Source: CAD feature listing. Evaluate the final solid. Frame: model axes, mm. Face numbers are marked on the shaded views. Give positions to 0.01 mm unless a question says otherwise; leave off trailing zeros. Order: outer loops, then holes, each group sorted by start corner. A loop starts at its lowest first (then second) coordinate and runs counter-clockwise, first axis right, second up. Notation, with made-up numbers: (10, -4.75) -> (20, -4.75) arc R21 cw to (20, 4.25) -> close; hole circle Ø4 at (-36, 58.5). An arc over 180 degrees is marked (long way). Answer in a Markdown table with one row per item.
```python
from build123d import *

# Parameters (mm, degrees)
BOSS_EXTRUDE1_DEPTH = 20
SKETCH2_R           = 10
CUT_EXTRUDE1_DEPTH  = 20


with BuildPart() as part:
    # Sketch1 → Boss-Extrude1 (new body)
    with BuildSketch(Plane.XY):
        Polygon((-19.976319314, 0), (-9.988159657, -17.3), (9.988159657, -17.3), (19.976319314, 0), (9.988159657, 17.3), (-9.988159657, 17.3), align=None)
    extrude(amount=BOSS_EXTRUDE1_DEPTH)

    # Sketch2 → Cut-Extrude1 (cut)
    with BuildSketch(Plane.XY.offset(20)):
        Circle(SKETCH2_R)
    extrude(amount=-CUT_EXTRUDE1_DEPTH, mode=Mode.SUBTRACT)

    # Sketch3 → Cut-Revolve1 (revolve, cut)
    with BuildSketch(Plane(origin=(0, 0, 0), x_dir=(1, 0, 0), z_dir=(0, 1, 0))):
        with BuildLine():
            Line((19.976319314, -2), (19.976319314, 0))
            Line((19.976319314, 0), (17.976319314, 0))
            ThreePointArc((17.976319314, 0), (19.390532876, -0.585786438), (19.976319314, -2))
        make_face()
    cut_revolve1 = revolve(axis=Axis((0, 0, 0), (0, 0, 1)), mode=Mode.SUBTRACT)

    # Mirror1: Cut-Revolve1 across plane
    add(cut_revolve1.mirror(Plane(origin=(0, 0, 10), x_dir=(1, 0, 0), z_dir=(0, 0, -1))), mode=Mode.SUBTRACT)


solid = part.part
```
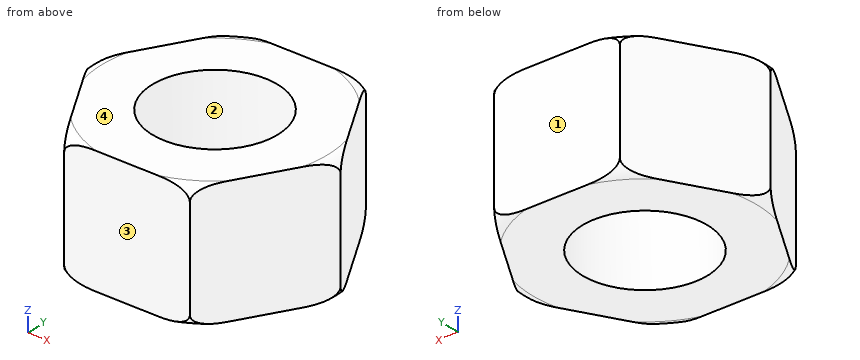
(1) Ray query, probe 1 along Y at (x, z) = (0, 14); probe 2 along Y at (x, z) = (-8.5, 6); probe 3 along X at (y, z) = (-4.5, 9.25). Return the intervals inside material, ascending.
A:
| item | result |
|---|---|
| probe 1 | y = -17.3 to -10, 10 to 17.3 |
| probe 2 | y = -17.3 to -5.27, 5.27 to 17.3 |
| probe 3 | x = -17.38 to -8.93, 8.93 to 17.38 |
(2) Section query D-D (z = 18.5). Return the cut outline in (x, y), plus the area to 3 significant figures.
A:
| item | result |
|---|---|
| outline | (-19.91, -0.11) -> (-10.05, -17.19) arc R19.91 ccw to (-9.86, -17.3) -> (9.86, -17.3) arc R19.91 ccw to (10.05, -17.19) -> (19.91, -0.11) arc R19.91 ccw to (19.91, 0.11) -> (10.05, 17.19) arc R19.91 ccw to (9.86, 17.3) -> (-9.86, 17.3) arc R19.91 ccw to (-10.05, 17.19) -> (-19.91, 0.11) arc R19.91 ccw to start; hole circle Ø20 at (0, 0) |
| area | 723 mm^2 |
(3) Pull-direction query (Y, two-part tool) for the marked faces 1, 2, 3 and 4; classes: +Y half, -Y half, draft (parallel to the pull), parting line (faces both ways), or undercut.
A:
| item | result |
|---|---|
| face 1 | +Y half |
| face 2 | undercut |
| face 3 | -Y half |
| face 4 | draft |
(4) Section query A-A (x = 0). Return the cut outline in (y, z).
A:
| item | result |
|---|---|
| outline | (-17.3, 0) -> (-10, 0) -> (-10, 20) -> (-17.3, 20) -> close; (10, 0) -> (17.3, 0) -> (17.3, 20) -> (10, 20) -> close |
(5) Section query C-C (y = 9.5). Return the cut outline in (x, z).
A:
| item | result |
|---|---|
| outline | (-14.49, 0) -> (-3.12, 0) -> (-3.12, 20) -> (-14.49, 20) -> close; (3.12, 0) -> (14.49, 0) -> (14.49, 20) -> (3.12, 20) -> close |
(6) Section query B-B (z = 16.25). Return the cut outline in (x, y), plus the area to 3 significant figures.
A:
| item | result |
|---|---|
| outline | (-19.98, 0) -> (-9.99, -17.3) -> (9.99, -17.3) -> (19.98, 0) -> (9.99, 17.3) -> (-9.99, 17.3) -> close; hole circle Ø20 at (0, 0) |
| area | 723 mm^2 |
(7) First-contact query: pin 1 Ø4 at (y, z) = (9, 8.5) entering from -X; pin 2 Ø2 at (y, z) = (4.5, 8) entering from +X. Flat tips, straight axial feed; report the tip coordinate or a pass-through.
A:
| item | result |
|---|---|
| pin 1 | stops at x = -15.93 |
| pin 2 | stops at x = 17.96 |
